```python
from build123d import *

# Parameters (mm, degrees)
SKETCH1_W           = 54
SKETCH1_H           = 50
SKETCH1_R           = 23.9
BOSS_EXTRUDE1_DEPTH = 68.2
SKETCH2_W           = 54
SKETCH2_H           = 50
SKETCH2_R           = 16
BOSS_EXTRUDE2_DEPTH = 2
LPATTERN1_COUNT     = 2
LPATTERN1_PITCH     = 70.2
SKETCH3_R           = 2
CUT_EXTRUDE1_DEPTH  = 7
BOSS_EXTRUDE5_START = 2
SKETCH7_W           = 54
SKETCH7_H           = 50
SKETCH7_R           = 16
BOSS_EXTRUDE5_DEPTH = 2
SKETCH6_W           = 54
SKETCH6_H           = 50
SKETCH6_R           = 16
BOSS_EXTRUDE6_DEPTH = 2
SKETCH8_R           = 23.9
CUT_EXTRUDE2_DEPTH  = 0.25
CUT_EXTRUDE3_START  = -0.25
SKETCH9_R           = 23.9
CUT_EXTRUDE3_DEPTH  = 0.25
SKETCH10_W          = 9
SKETCH10_H          = 50
CUT_EXTRUDE4_DEPTH  = 2.1
SKETCH11_W          = 9
SKETCH11_H          = 50
CUT_EXTRUDE5_DEPTH  = 2.1


with BuildPart() as part:
    # Sketch1 → Boss-Extrude1 (new body)
    with BuildSketch(Plane(origin=(0, 0, 0), x_dir=(0, 0, -1), z_dir=(1, 0, 0))):
        Rectangle(SKETCH1_W, SKETCH1_H)
        Circle(SKETCH1_R, mode=Mode.SUBTRACT)
    extrude(amount=BOSS_EXTRUDE1_DEPTH)

    # Sketch2 → Boss-Extrude2 (add)
    with BuildSketch(Plane(origin=(68.2, 0, 0), x_dir=(0, 0, -1), z_dir=(1, 0, 0))):
        Rectangle(SKETCH2_W, SKETCH2_H)
        Circle(SKETCH2_R, mode=Mode.SUBTRACT)
    boss_extrude2 = extrude(amount=BOSS_EXTRUDE2_DEPTH)

    # LPattern1: Boss-Extrude2 ×2
    with Locations(*[(-i * LPATTERN1_PITCH, 0, 0) for i in range(1, LPATTERN1_COUNT)]):
        add(boss_extrude2)

    # Sketch3 → Cut-Extrude1 (cut)
    with BuildSketch(Plane.XZ.offset(25)):
        with Locations(Location((3, 22, 0), (0, 0, 270))):
            Circle(SKETCH3_R)
        with Locations(Location((65.2, 22, 0), (0, 0, 270))):
            Circle(SKETCH3_R)
        with Locations(Location((65.2, -22, 0), (0, 0, 270))):
            Circle(SKETCH3_R)
        with Locations(Location((3, -22, 0), (0, 0, 270))):
            Circle(SKETCH3_R)
    cut_extrude1 = extrude(amount=-CUT_EXTRUDE1_DEPTH, mode=Mode.SUBTRACT)

    # Mirror1: Cut-Extrude1 across plane
    add(cut_extrude1.mirror(Plane.ZX), mode=Mode.SUBTRACT)

    # Sketch7 → Boss-Extrude5 (add)
    with BuildSketch(Plane.ZY.offset(2).offset(BOSS_EXTRUDE5_START)):
        Rectangle(SKETCH7_W, SKETCH7_H)
        with Locations(Location((0, 0, 0), (0, 0, 180))):
            Circle(SKETCH7_R, mode=Mode.SUBTRACT)
    extrude(amount=-BOSS_EXTRUDE5_DEPTH)

    # Sketch6 → Boss-Extrude6 (add)
    with BuildSketch(Plane(origin=(70.2, 0, 0), x_dir=(0, 0, -1), z_dir=(1, 0, 0))):
        Rectangle(SKETCH6_W, SKETCH6_H)
        Circle(SKETCH6_R, mode=Mode.SUBTRACT)
    extrude(amount=BOSS_EXTRUDE6_DEPTH)

    # Sketch8 → Cut-Extrude2 (cut)
    with BuildSketch(Plane.ZY.offset(-68.2)):
        Circle(SKETCH8_R)
    extrude(amount=-CUT_EXTRUDE2_DEPTH, mode=Mode.SUBTRACT)

    # Sketch9 → Cut-Extrude3 (cut)
    with BuildSketch(Plane(origin=(0, 0, 0), x_dir=(0, 0, -1), z_dir=(1, 0, 0)).offset(CUT_EXTRUDE3_START)):
        with Locations(Location((0, 0, 0), (0, 0, 180))):
            Circle(SKETCH9_R)
    extrude(amount=CUT_EXTRUDE3_DEPTH, mode=Mode.SUBTRACT)

    # Sketch10 → Cut-Extrude4 (cut)
    with BuildSketch(Plane(origin=(72.2, 0, 0), x_dir=(0, 0, -1), z_dir=(1, 0, 0))):
        with Locations((-22.5, 0)):
            Rectangle(SKETCH10_W, SKETCH10_H)
        with Locations((22.5, 0)):
            Rectangle(SKETCH10_W, SKETCH10_H)
    extrude(amount=-CUT_EXTRUDE4_DEPTH, mode=Mode.SUBTRACT)

    # Sketch11 → Cut-Extrude5 (cut)
    with BuildSketch(Plane.ZY.offset(4)):
        with Locations((-22.5, 0)):
            Rectangle(SKETCH11_W, SKETCH11_H)
        with Locations((22.5, 0)):
            Rectangle(SKETCH11_W, SKETCH11_H)
    extrude(amount=-CUT_EXTRUDE5_DEPTH, mode=Mode.SUBTRACT)


solid = part.part
```
Build history of the part. All positions in model axes, mm. A direction names the side the tool comes from. Round coordinates to 2 decimals unless told otherwise and drop trailing zeros. Loops run counter-clockwise (first coordinate to the right, second up) from the corner with the lowest first, then second, coordinate; pieces in that order, holes last. Notation, with made-up numbers: M 23.5,-1 L 47.5,-1 A15 ccw 47.5,22 Z; hole C -6,80 d1. An arc over 180 degrees is marked long. Answer as CSV lines item,"result".
1. Cut at B-B on z = 2. Write the cut outline in (x, y).
Resolved:
outline,"M -4,-25 L 72.2,-25 L 72.2,-15.87 L 68.45,-15.87 L 68.45,-23.82 L -0.25,-23.82 L -0.25,-15.87 L -4,-15.87 Z; M -4,15.87 L -0.25,15.87 L -0.25,23.82 L 68.45,23.82 L 68.45,15.87 L 72.2,15.87 L 72.2,25 L -4,25 Z"
2. Cut at C-C on x = 3. Write the cut outline in (y, z), then the cut area to 3 significant figures.
Resolved:
outline,"M -25,-27 L 25,-27 L 25,-24 L 18,-24 L 18,-20 L 25,-20 L 25,20 L 18,20 L 18,24 L 25,24 L 25,27 L -25,27 L -25,24 L -18,24 L -18,20 L -25,20 L -25,-20 L -18,-20 L -18,-24 L -25,-24 Z; hole C 0,0 d47.8"
area,"793 mm²"
3. Wall check: probe 1 along X at (y, z) = (-22, 22); probe 2 along Y at (x, z) = (-1.65, 0); probe 3 along X at (y, z) = (13, 9.5). Give the ranges that are in metal, low to high. Write a range as [from, to].
Resolved:
probe 1,"x = [-1.9, 1], [5, 63.2], [67.2, 70.1]"
probe 2,"y = [-25, -16], [16, 25]"
probe 3,"x = [-4, -0.25], [68.45, 72.2]"
4. Cut at A-A on y = 0. Write the cut outline in (x, z).
Resolved:
outline,"M -4,-18 L -1.9,-18 L -1.9,-27 L 70.1,-27 L 70.1,-18 L 72.2,-18 L 72.2,-16 L 68.45,-16 L 68.45,-23.9 L -0.25,-23.9 L -0.25,-16 L -4,-16 Z; M -4,16 L -0.25,16 L -0.25,23.9 L 68.45,23.9 L 68.45,16 L 72.2,16 L 72.2,18 L 70.1,18 L 70.1,27 L -1.9,27 L -1.9,18 L -4,18 Z"
5. Cut at D-D on z = -22. Write the cut outline in (x, y), then the cut area to 3 significant figures.
Resolved:
outline,"M -1.9,-25 L 1,-25 L 1,-18 L 5,-18 L 5,-25 L 63.2,-25 L 63.2,-18 L 67.2,-18 L 67.2,-25 L 70.1,-25 L 70.1,25 L 67.2,25 L 67.2,18 L 63.2,18 L 63.2,25 L 5,25 L 5,18 L 1,18 L 1,25 L -1.9,25 Z; hole M -0.25,-9.34 L 68.45,-9.34 L 68.45,9.34 L -0.25,9.34 Z"
area,"2,200 mm²"
6. 3-axis set-ups, long thin cutter, end or side, ignore diameter. For faces 1 (the cylindrical face through (1.8, -21.5, 23.6)), 2 (the flat face through (70.1, 0, -22)), 3 (the cylindrical face through (66.886, 21.549, -23.075)): which of +Z, -Z, +X, -X, +Y, -Y reach the whole face in a straight line?
Resolved:
face 1,"-Y"
face 2,"-Z, +X, +Y, -Y"
face 3,"+Y"
7. Two-plate mould, pull along Z, no slides. Class faces 4 (the flat face through (-4, 0.4, -16.3)), 5 (the flat face through (65, 18, -22)), 6 (the flat face through (71, 0, -18)): released by +Z, released by -Z, zero draft, split by the parting line, or undercut.
Resolved:
face 4,"zero draft"
face 5,"undercut"
face 6,"released by -Z"
8. Flat gauge pins, fed straight in: P1, Ø0.6, axis at x = -2.5, y = 0, coming from the -Z side; P2, Ø2.5, axis at x = 65.2, z = -22, coming from the -Y side; P3, Ø6, axis at y = 10, z = 7, coming from the +X side; P4, Ø3.5, axis at x = 3, z = -22, coming from the +Y side. Where does each tip first touch, or does it go through?
Resolved:
P1,"stops at z = -18"
P2,"stops at y = -18"
P3,"passes through"
P4,"stops at y = 18"
